For this review, take the finished solid that the model builds, in its own axes (mm). A direction names the side the tool comes from. Give positions to 0.01 mm unless a question says otherwise; leave off trailing zeros. Order: outer loops, then holes, each group sorted by start corner. A loop starts at its lowest first (then second) coordinate and runs counter-clockwise, first axis right, second up. Notation, with made-up numbers: (32, 53) - (83, 53) arc R24 cw to (83, 72) - close; hole circle Ø8 at (-37.5, -8). An arc over 180 degrees is marked (long way). One line per item, written item: value.
Autodesk Inventor part; units mm, degrees
ref_plane "YZ Plane" through (0, 0, 0) normal (1, 0, 0) x (0, 1, 0)
ref_plane "XZ Plane" through (0, 0, 0) normal (0, 1, 0) x (-1, 0, 0)
ref_plane "XY Plane" through (0, 0, 0) normal (0, 0, 1) x (1, 0, 0)
sketch "Sketch1" plane through (0, 0, 0) normal (0, 0, 1) x (1, 0, 0)
  circle A0 centre (0, 0) radius 3
  dimension "d0" = 6
extrude "Extrusion1" add sketch "Sketch1" along normal blind 150
sketch "Sketch2" plane through (0, 0, 150) normal (0, 0, 1) x (1, 0, 0)
  circle A0 centre (0, 0) radius 8
  dimension "d3" = 16
extrude "Extrusion2" add sketch "Sketch2" along normal blind 20
sketch "Sketch3" plane through (0, 0, 0) normal (1, 0, 0) x (0, 1, 0)
  circle A0 centre (0, 160) radius 3
  point P0 (0, 0)
  dimension "d6" = 6
extrude "Extrusion3" cut sketch "Sketch3" along normal mid plane 20
properties part number "ana_vida_mili"
(1) Wall thickness on line 1 (Z direction, x = 3.5, y = 0); line 2 (Z direction, x = 2.75, y = 3.75); line 3 (Z direction, x = 0, y = 2.75): over which ranges is each line inside the solid? List them lowest first. Write a range as from..to.
Answers below:
line 1: z = 150..157, 163..170
line 2: z = 150..170
line 3: z = 0..158.8, 161.2..170
(2) Take a section at A-A (x = 0). Write out the cut boundary in (y, z), then the cut area to 3 significant figures.
Answers below:
outline: (-8, 150) - (-3, 150) - (-3, 0) - (3, 0) - (3, 150) - (8, 150) - (8, 170) - (-8, 170) - close; hole circle Ø6 at (0, 160)
area: 1,190 mm^2
(3) Take a section at D-D (z = 90.5). Write out the cut boundary in (x, y).
Answers below:
outline: circle Ø6 at (0, 0)
(4) For P1, Ø4, axis at x = 2.5, z = 121.5, coming from the -Y side; P2, Ø1, axis at y = -4, z = 62, coming from the -X side; P3, Ø5, axis at y = -6, z = 148.5, coming from the +X side, all flat-tipped, find the tip position at first contact; note any pin that passes through.
Answers below:
P1: stops at y = -2.96
P2: passes through
P3: stops at x = 6.93
(5) Machinability: for faces 4 (the face through (0, 0, 0)), 5 (the face through (3.4, 0.1, 150)), which of the approach directions +Z, -Z, +X, -X, +Y, -Y give a long, thin tool a straight path to every point of the face, cutting with its end or side? Answer none if there is none.
Answers below:
face 4: -Z, +X, -X, +Y, -Y
face 5: -Z
(6) Draft analysis for pull direction Y (two halves, no side actions). For faces 1 (the face through (3.69, 7.1, 159.86)), 2 (the face through (-0.11, 1.61, 157.47)), 3 (the face through (0, 0, 170)), state which applies: pulls with the +Y half, pulls with the -Y half, needs draft (parallel to the pull), parting line crosses it, or undercut.
Answers below:
face 1: parting line crosses it
face 2: undercut
face 3: needs draft
(7) Take a section at B-B (y = -1.5). Write out the cut boundary in (x, z), then the cut area to 3 significant figures.
Answers below:
outline: (-7.86, 150) - (-2.6, 150) - (-2.6, 0) - (2.6, 0) - (2.6, 150) - (7.86, 150) - (7.86, 157.4) - (-7.86, 157.4) - close; (-7.86, 162.6) - (7.86, 162.6) - (7.86, 170) - (-7.86, 170) - close
area: 1,010 mm^2
(8) Take a section at C-C (z = 160). Write out the cut boundary in (x, y), then the cut area to 3 significant figures.
Answers below:
outline: (-7.42, -3) arc R8 ccw to (7.42, -3) - close; (-7.42, 3) - (7.42, 3) arc R8 ccw to start
area: 107 mm^2
